Source: CAD feature listing. Evaluate the final solid. Frame: model axes, mm. A direction names the side the tool comes from. Give positions to 0.01 mm unless a question says otherwise; leave off trailing zeros. Loops run counter-clockwise (first coordinate to the right, second up) from the corner with the lowest first, then second, coordinate; pieces in that order, holes last. Notation, with made-up numbers: (57, 61) -> (62, 61) arc R10 cw to (62, 68) -> close; hole circle Ø7 at (84, 24). An arc over 180 degrees is marked (long way). Return JSON: item names as keys, results as strings. Group by question number.
(1) Access query for faces 4 (the face through (-2, -4, 3)), 5 (the face through (1.08, -4.88, -0.49)). Directions: +Z, -Z, +X, -X, +Y, -Y. A direction counts if a zero-diameter tool reaches every point of the face in a straight line with its end or side. Return the directions, or none.
(2) Pin query (flat end, axial travel): pin 1 (1 mm diameter, centred on x = -1.5, y = -2.5, fed in from +Z). Return the tip coordinate at first contact, or that it passes through.
(3) Ray query, line 1 (Y direction, x = 0, z = 1.4) (3 decimals); line 2 (Z direction, x = -2, y = -7); line 3 (Y direction, x = 0.5, z = 2.2). Return the intervals inside material, ascending. Write a range as from..to.
(4) Cut plane C-C on z = 2.3. Return loops of the section in (x, y) (3 decimals).
(5) Cut plane D-D on x = -4.25. Return loops of the section in (y, z).
(6) Draft query along X for faces 1 (the face through (7.874, 2.48, 1.479)), 2 (the face through (0.867, -3.905, 0.972)), 3 (the face through (4, -4, 0)). Return one class per face: released by +X, released by -X, zero draft, split by the parting line, or undercut.
(7) Cut plane A-A on x = 0. Return loops of the section in (y, z) (3 decimals).
```python
from build123d import *

# Parameters (mm, degrees)
SKETCH1_R           = 8.255
BOSS_EXTRUDE1_DEPTH = 3
SKETCH2_R           = 5
BOSS_EXTRUDE2_DEPTH = 1
SKETCH3_R           = 4
CUT_EXTRUDE1_DEPTH  = 5


with BuildPart() as part:
    # Sketch1 → Boss-Extrude1 (new body)
    with BuildSketch(Plane.XY):
        Circle(SKETCH1_R)
    extrude(amount=BOSS_EXTRUDE1_DEPTH)

    # Sketch2 → Boss-Extrude2 (add)
    with BuildSketch(Plane(origin=(0, 0, 0), x_dir=(-1, 0, 0), z_dir=(0, 0, -1))):
        Circle(SKETCH2_R)
    extrude(amount=BOSS_EXTRUDE2_DEPTH)

    # Sketch3 → Cut-Extrude1 (cut, through all)
    with BuildSketch(Plane(origin=(0, 0, -1), x_dir=(-1, 0, 0), z_dir=(0, 0, -1))):
        Circle(SKETCH3_R)
    extrude(amount=-CUT_EXTRUDE1_DEPTH, mode=Mode.SUBTRACT)


solid = part.part
```
Answers:
{
 "1": {"face 4": "+Z, +X, -X, +Y, -Y", "face 5": "-Z"},
 "2": {"pin 1": "through"},
 "3": {"line 1": "-8.255..-4, 4..8.255", "line 2": "0..3", "line 3": "-8.24..-3.97, 3.97..8.24"},
 "4": {"outline": "circle Ø16.51 at (0, 0); hole circle Ø8 at (0, 0)"},
 "5": {"outline": "(-7.08, 0) -> (-2.63, 0) -> (-2.63, -1) -> (2.63, -1) -> (2.63, 0) -> (7.08, 0) -> (7.08, 3) -> (-7.08, 3) -> close"},
 "6": {"face 1": "split by the parting line", "face 2": "undercut", "face 3": "zero draft"},
 "7": {"outline": "(-8.255, 0) -> (-5, 0) -> (-5, -1) -> (-4, -1) -> (-4, 3) -> (-8.255, 3) -> close; (4, -1) -> (5, -1) -> (5, 0) -> (8.255, 0) -> (8.255, 3) -> (4, 3) -> close"}
}
